Read the model definition and answer for the solid it produces. Units are mm, in the model's axes. Face numbers are marked on the shaded views. Give positions to 0.01 mm unless a question says otherwise; leave off trailing zeros. Order: outer loops, then holes, each group sorted by start corner. A loop starts at its lowest first (then second) coordinate and runs counter-clockwise, first axis right, second up. Notation, with made-up numbers: (-28.75, -9) -> (30.25, -9) arc R15 ccw to (30.25, 20) -> close; hole circle Ø10 at (32.5, -39.5). An arc over 180 degrees is marked (long way). One line per item, written item: value. Start each with the question number.
from build123d import *

# Parameters (mm, degrees)
SKETCH_1_R      = 12.5
EXTRUDE_1_DEPTH = 15
SKETCH_2_R      = 22.5
SKETCH_2_R_2    = 1
EXTRUDE_2_DEPTH = 2
SKETCH_3_R      = 22.5
EXTRUDE_3_DEPTH = 2


with BuildPart() as part:
    # 草图1 → 凸台-拉伸1 (new body)
    with BuildSketch(Plane(origin=(0, 0, 0), x_dir=(1, 0, 0), z_dir=(0, 1, 0))):
        with Locations(Location((0, 0, 0), (0, 0, 270))):
            Circle(SKETCH_1_R)
        with BuildLine():
            Line((-1.469693846, -1.5), (1.469693846, -1.5))
            ThreePointArc((1.469693846, -1.5), (0, 2.1), (-1.469693846, -1.5))
        make_face(mode=Mode.SUBTRACT)
    extrude(amount=EXTRUDE_1_DEPTH)

    # 草图2 → 凸台-拉伸2 (add)
    with BuildSketch(Plane.XZ):
        with Locations(Location((0, 0, 0), (0, 0, 270))):
            Circle(SKETCH_2_R)
        with Locations(Location((0, 20, 0), (0, 0, 270))):
            Circle(SKETCH_2_R_2, mode=Mode.SUBTRACT)
        with Locations(Location((5.176380902, 19.318516526, 0), (0, 0, 270))):
            Circle(SKETCH_2_R_2, mode=Mode.SUBTRACT)
        with BuildLine():
            Line((-1.469693846, 1.5), (1.469693846, 1.5))
            ThreePointArc((1.469693846, 1.5), (0, -2.1), (-1.469693846, 1.5))
        make_face(mode=Mode.SUBTRACT)
    extrude(amount=-EXTRUDE_2_DEPTH)

    # 草图3 → 凸台-拉伸3 (add)
    with BuildSketch(Plane(origin=(0, 15, 0), x_dir=(1, 0, 0), z_dir=(0, 1, 0))):
        with Locations(Location((0, 0, 0), (0, 0, 90))):
            Circle(SKETCH_3_R)
        with BuildLine():
            Line((-1.469693846, -1.5), (1.469693846, -1.5))
            ThreePointArc((1.469693846, -1.5), (0, 2.1), (-1.469693846, -1.5))
        make_face(mode=Mode.SUBTRACT)
    extrude(amount=EXTRUDE_3_DEPTH)


solid = part.part
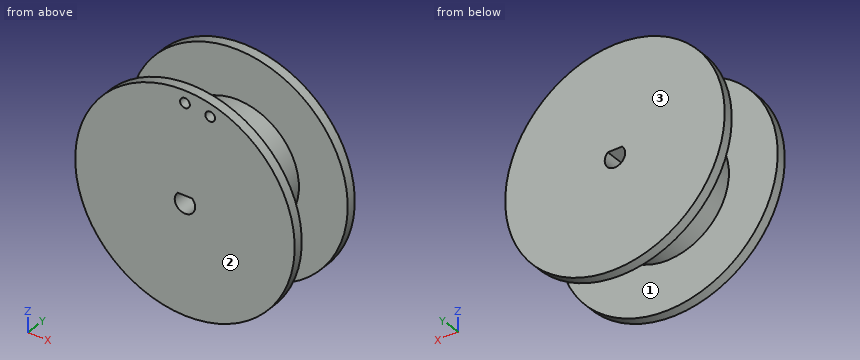
Item 1: For a pull along Y with two mould halves and no side action, classify the marked faces 1, 2 and 3 as +Y half, -Y half, draft (parallel to the pull), parting line (faces both ways), or undercut.
Item 2: Find section D-D on y = 4.5. Write down the section's boundary in (x, z), then the cut area to 3 significant figures.
Item 3: Flat-ended cylindrical pins translate along their axes: pin 1 (5 mm diameter, centred on y = 11.5, z = 5.5, fed in from +X); pin 2 (5 mm diameter, centred on y = 12, z = -10.5, fed in from -X); pin 3 (4 mm diameter, centred on y = 3.5, z = 13.5, fed in from +X); pin 4 (8 mm diameter, centred on y = 9, z = 17.5, fed in from +X). Find the tip coordinate at first contact, or state that the pin passes through.
Item 4: Find section C-C on z = 0. Write down the section's boundary in (x, y).
Item 5: Find section B-B on x = 0. Write down the section's boundary in (y, z).
Item 6: Find section A-A on x = 13.5. Write down the section's boundary in (y, z), then the cut area to 3 significant figures.
Item 7: Find the intervals of material crossed by line 1 (X direction, y = 13, z = 0); line 2 (Y direction, x = -13, z = -11.5); line 3 (Z direction, x = 0, y = 9.75), in increasing order. Write a range as from..to.
Checks:
1. face 1: undercut
1. face 2: -Y half
1. face 3: +Y half
2. outline: circle Ø25 at (0, 0); hole (-1.47, 1.5) arc R2.1 ccw (long way) to (1.47, 1.5) -> close
2. area: 478 mm2
3. pin 1: x = 12.13
3. pin 2: x = -9.6
3. pin 3: x = 18.92
3. pin 4: through
4. outline: (-22.5, 0) -> (-2.1, 0) -> (-2.1, 17) -> (-22.5, 17) -> (-22.5, 15) -> (-12.5, 15) -> (-12.5, 2) -> (-22.5, 2) -> close; (2.1, 0) -> (22.5, 0) -> (22.5, 2) -> (12.5, 2) -> (12.5, 15) -> (22.5, 15) -> (22.5, 17) -> (2.1, 17) -> close
5. outline: (0, -22.5) -> (2, -22.5) -> (2, -12.5) -> (15, -12.5) -> (15, -22.5) -> (17, -22.5) -> (17, -2.1) -> (0, -2.1) -> close; (0, 1.5) -> (17, 1.5) -> (17, 22.5) -> (15, 22.5) -> (15, 12.5) -> (2, 12.5) -> (2, 19) -> (0, 19) -> close; (0, 21) -> (2, 21) -> (2, 22.5) -> (0, 22.5) -> close
6. outline: (0, -18) -> (2, -18) -> (2, 18) -> (0, 18) -> close; (15, -18) -> (17, -18) -> (17, 18) -> (15, 18) -> close
6. area: 144 mm2
7. line 1: -12.5..-2.1, 2.1..12.5
7. line 2: 0..2, 15..17
7. line 3: -12.5..-2.1, 1.5..12.5
